Design review of the part built by this model. Coordinates are the model's own, in mm. A direction names the side the tool comes from. Give positions to 0.01 mm unless a question says otherwise; leave off trailing zeros. Order: outer loops, then holes, each group sorted by start corner. A loop starts at its lowest first (then second) coordinate and runs counter-clockwise, first axis right, second up. Notation, with made-up numbers: (-19, 22) -> (38, 22) arc R22 cw to (38, 35) -> close; hole circle Ø9 at (42.5, -20). An arc over 180 degrees is marked (long way). Use a Markdown table: item, result. Add a question column.
```python
from build123d import *

# Parameters (mm, degrees)
BOSS_EXTRUDE2_DEPTH     = 8
SKETCH2_R               = 1.6
CUT_EXTRUDE1_DEPTH      = 8
SKETCH3_R               = 5
BOSS_EXTRUDE3_DEPTH     = 12
CUT_EXTRUDE3_DEPTH      = 43.5
CUT_EXTRUDE3_DEPTH_BACK = 43.5


with BuildPart() as part:
    # Sketch1 → Boss-Extrude2 (new body)
    with BuildSketch(Plane.XY):
        with BuildLine():
            Line((0, 0), (-15, 0))
            Line((-15, 0), (-15, 5))
            Line((-15, 5), (-7, 5))
            Line((-7, 5), (-7, 17.5))
            ThreePointArc((-7, 17.5), (-5.535533906, 21.035533906), (-2, 22.5))
            Line((-2, 22.5), (2, 22.5))
            ThreePointArc((2, 22.5), (5.535533906, 21.035533906), (7, 17.5))
            Line((7, 17.5), (7, 5))
            Line((7, 5), (15, 5))
            Line((15, 5), (15, 0))
            Line((15, 0), (0, 0))
        make_face()
    extrude(amount=BOSS_EXTRUDE2_DEPTH)

    # Sketch2 → Cut-Extrude1 (cut)
    with BuildSketch(Plane(origin=(0, 5, 0), x_dir=(1, 0, 0), z_dir=(0, 1, 0))):
        with Locations(Location((-11, -4, 0), (0, 0, 270))):
            Circle(SKETCH2_R)
        with Locations(Location((11, -4, 0), (0, 0, 180))):
            Circle(SKETCH2_R)
    extrude(amount=-CUT_EXTRUDE1_DEPTH, mode=Mode.SUBTRACT)

    # Sketch3 → Boss-Extrude3 (add)
    with BuildSketch(Plane.XY.offset(8)):
        with Locations((0, 14.5)):
            Circle(SKETCH3_R)
    extrude(amount=BOSS_EXTRUDE3_DEPTH)

    # Sketch8 → Cut-Extrude3 (cut, two sides: drawn at the far end of the back side and taken through both)
    with BuildSketch(Plane.ZY.offset(15).offset(-CUT_EXTRUDE3_DEPTH_BACK)):
        Polygon((-14.53213237, -58.578079117), (0, 5), (4, 22.5), (18.53213237, 86.078079117), (-108.624025864, 115.142343856), (-141.688290603, -29.513814378), align=None)
    extrude(amount=CUT_EXTRUDE3_DEPTH + CUT_EXTRUDE3_DEPTH_BACK, mode=Mode.SUBTRACT)


solid = part.part
```
1) The part is to be moulded in two halves that separate along X. For faces 1 (the cylindrical face through (12.6, 2.54, 4.07)), 2 (the flat face through (0, 9, 8)), 3 (the cylindrical face through (-1.08, 9.62, 13.92)), 4 (the cylindrical face through (-12.42, 2.54, 4.74)), say which applies: +X half, -X half, draft (parallel to the pull), parting line (faces both ways), or undercut.
2) Insertion check: pin 1 (6.5 mm diameter, centred on x = 9, z = 2.5, fed in from +Y); pin 2 (4 mm diameter, centred on x = -4.5, z = 12, fed in from -Y); pin 3 (5 mm diameter, centred on x = -6, y = 5.5, fed in from -Z); pin 4 (6 mm diameter, centred on x = -2.5, y = 16, fed in from -Z). Each pin has a flat end and moves straight along its axis. Give the tip position at first contact, or say it passes through.
3) Add section A-A (x = 11). Give the boundary of the cut face in (y, z), then the cut area to 3 significant figures.
4) Add section D-D (y = 10.5). Give the boundary of the cut face in (x, z), then the cut area to 3 significant figures.
5) Add section B-B (y = 14). Give the boundary of the cut face in (x, z), then the cut area to 3 significant figures.
6) For L1, parallel to Y at x = -10.5, z = 1.5; L2, parallel to Z at x = -2, y = 5.25; L3, parallel to Y at x = -0.5, z = 9.75, list the stretches that pass through material, from the lowest coordinate up. Write a range as [from, to].
7) Machinability: for faces 5 (the flat face through (-7, 11, 5)), 6 (the flat face through (7, 11, 5)), 7 (the flat face through (15, 3, 4)), which of the approach directions +Z, -Z, +X, -X, +Y, -Y give a long, thin tool a straight path to every point of the face, cutting with its end or side? Answer none if there is none.
8) Add section C-C (x = 0). Give the boundary of the cut face in (y, z), then the cut area to 3 significant figures.
Worked answers:
| question | item | result |
|---|---|---|
| 1 | face 1 | undercut |
| 1 | face 2 | draft |
| 1 | face 3 | parting line |
| 1 | face 4 | undercut |
| 2 | pin 1 | y = 20.59 |
| 2 | pin 2 | y = 10.17 |
| 2 | pin 3 | z = 0 |
| 2 | pin 4 | z = 1.83 |
| 3 | outline | (0, 0) -> (5, 0) -> (5, 2.4) -> (0, 2.4) -> close; (0, 5.6) -> (5, 5.6) -> (5, 8) -> (0, 8) -> close |
| 3 | area | 24.0 mm^2 |
| 4 | outline | (-7, 1.26) -> (7, 1.26) -> (7, 8) -> (3, 8) -> (3, 20) -> (-3, 20) -> (-3, 8) -> (-7, 8) -> close |
| 4 | area | 166 mm^2 |
| 5 | outline | (-7, 2.06) -> (7, 2.06) -> (7, 8) -> (4.97, 8) -> (4.97, 20) -> (-4.97, 20) -> (-4.97, 8) -> (-7, 8) -> close |
| 5 | area | 203 mm^2 |
| 6 | L1 | [0, 5] |
| 6 | L2 | [0.06, 8] |
| 6 | L3 | [9.53, 19.47] |
| 7 | face 5 | +Z, -Z, -X, +Y |
| 7 | face 6 | +Z, -Z, +X, +Y |
| 7 | face 7 | +Z, -Z, +X, +Y, -Y |
| 8 | outline | (0, 0) -> (5, 0) -> (22.5, 4) -> (22.5, 8) -> (19.5, 8) -> (19.5, 20) -> (9.5, 20) -> (9.5, 8) -> (0, 8) -> close |
| 8 | area | 265 mm^2 |
